The drawing under review shows one solid part. Ordinate dimensions are in mm from its lowest x, y, z. A direction names the side the tool comes from. Round coordinates to 2 decimals unless told otherwise and drop trailing zeros. Loops run counter-clockwise (first coordinate to the right, second up) from the corner with the lowest first, then second, coordinate; pieces in that order, holes last. Notation, with made-up numbers: (-4.5, 44.25) - (49.5, 44.25) arc R11 cw to (49.5, 57.25) - close; hole circle Ø4 at (-29.5, 45.5). An arc over 180 degrees is marked (long way). Answer as CSV lines item,"result".
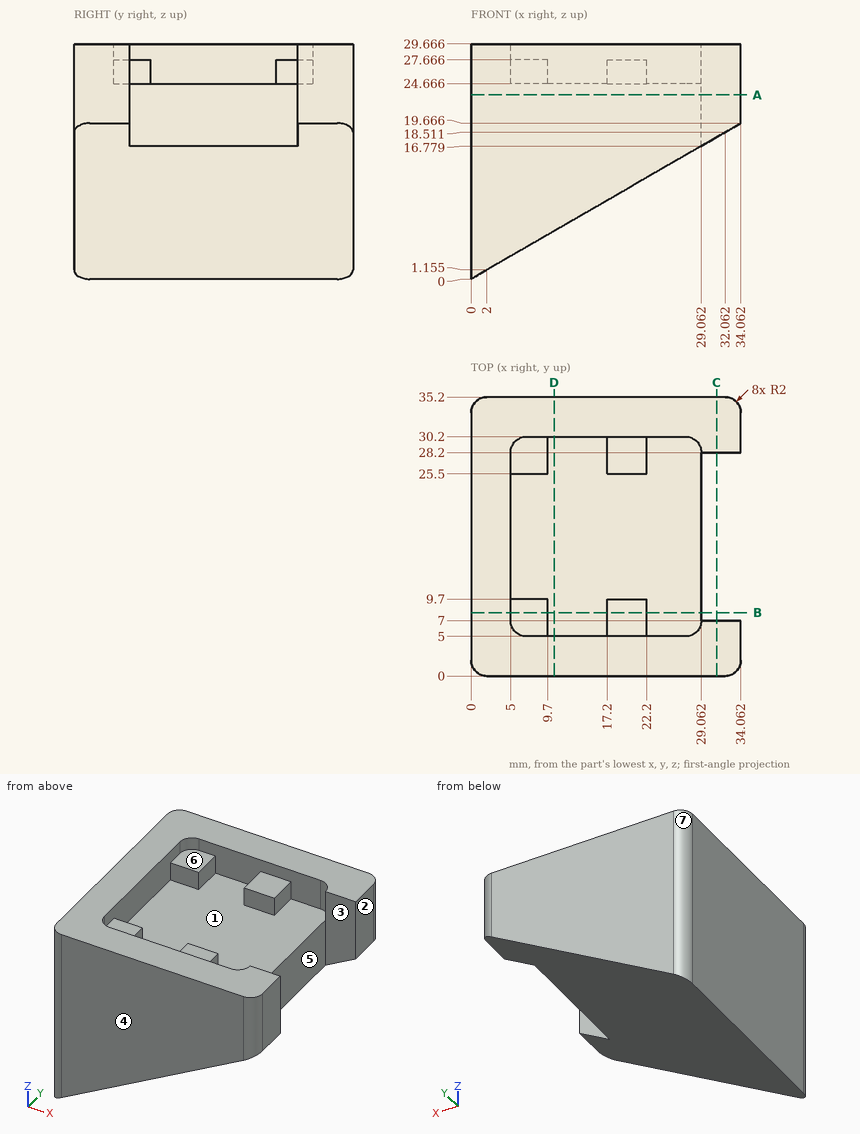
1. Take a section at B-B (y = 8). State the section outline as (x, z) points, plus the area to 3 significant figures.
Numbers:
outline,"(0, 0) - (29.06, 16.78) - (29.06, 24.67) - (22.2, 24.67) - (22.2, 27.67) - (17.2, 27.67) - (17.2, 24.67) - (9.7, 24.67) - (9.7, 27.67) - (5, 27.67) - (5, 29.67) - (0, 29.67) - close"
area,"527 mm²"
2. Take a section at C-C (x = 31). State the section outline as (y, z) points.
Numbers:
outline,"(0, 17.9) - (7, 17.9) - (7, 29.67) - (0, 29.67) - close; (28.2, 17.9) - (35.2, 17.9) - (35.2, 29.67) - (28.2, 29.67) - close"
3. Take a section at A-A (z = 23.25). State the section outline as (x, y) points.
Numbers:
outline,"(0, 2) arc R2 ccw to (2, 0) - (32.06, 0) arc R2 ccw to (34.06, 2) - (34.06, 7) - (29.06, 7) - (29.06, 28.2) - (34.06, 28.2) - (34.06, 33.2) arc R2 ccw to (32.06, 35.2) - (2, 35.2) arc R2 ccw to (0, 33.2) - close"
4. Clearance check with flat-ended pins moving along their axes: pin 1 (1.5 mm diameter, centred on y = 8.5, z = 26.5, fed in from +X); pin 2 (4 mm diameter, centred on y = 19.5, z = 22, fed in from +X); pin 3 (1 mm diameter, centred on x = 11, y = 26, fed in from -Z). State where each tip first meets the part, or that it passes through.
Numbers:
pin 1,"stops at x = 22.2"
pin 2,"stops at x = 29.06"
pin 3,"stops at z = 6.06"
5. Take a section at D-D (x = 10.5). State the section outline as (y, z) points, plus the area to 3 significant figures.
Numbers:
outline,"(0, 6.06) - (35.2, 6.06) - (35.2, 29.67) - (30.2, 29.67) - (30.2, 24.67) - (5, 24.67) - (5, 29.67) - (0, 29.67) - close"
area,"705 mm²"
6. Wall thickness on probe 1 along X at (y, z) = (12, 27); probe 2 along Y at (x, z) = (24, 26); probe 3 along X at (y, z) = (28.5, 28): over which ranges is each line inside the solid? List them lowest first.
Numbers:
probe 1,"x = 0 to 5"
probe 2,"y = 0 to 5, 30.2 to 35.2"
probe 3,"x = 0 to 5.02, 29.04 to 34.06"
7. Draft analysis for pull direction Y (two halves, no side actions). For the marked faces 1, 2, 3 and 4, state which applies: +Y half, -Y half, draft (parallel to the pull), parting line (faces both ways), or undercut.
Numbers:
face 1,"undercut"
face 2,"draft"
face 3,"undercut"
face 4,"-Y half"
8. Tool access review of the marked faces 5, 6 and 7: name each direction out of +Z, -Z, +X, -X, +Y, -Y from which nothing blocks a thin tool from reaching the whole face with its end or side.
Numbers:
face 5,"+Z, -Z, +X"
face 6,"+Z"
face 7,"+Z, -Z, -X, +Y"
